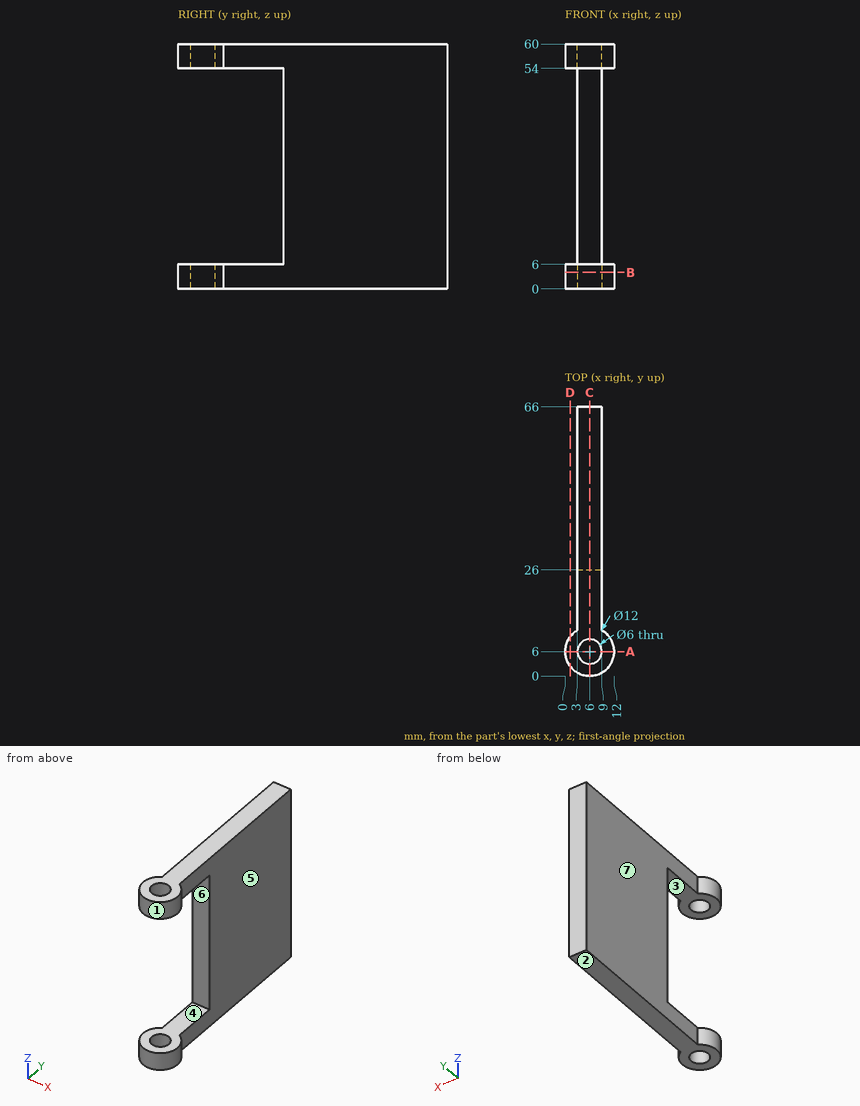
Geometry check sheet. Reference: drawing and pictorial views, mm from the part's lowest x, y, z. A direction names the side the tool comes from. Round coordinates to 2 decimals unless told otherwise and drop trailing zeros. Loops run counter-clockwise (first coordinate to the right, second up) from the corner with the lowest first, then second, coordinate; pieces in that order, holes last.
1. Sectioned sample at C-C on x = 6. Record the boundary of the cut face in (y, z), and give its area (3 significant figures).
2. Sectioned sample at B-B on z = 4. Record the boundary of the cut face in (x, y), and give its area (3 significant figures).
3. Set-up check for the marked faces 5, 6 and 7: record each of +Z, -Z, +X, -X, +Y, -Y from which the full face is reachable in a straight line by a thin tool's end or side.
4. Sectioned sample at A-A on y = 6. Record the boundary of the cut face in (x, z), and give its area (3 significant figures).
5. Sectioned sample at D-D on x = 1.25. Record the boundary of the cut face in (y, z).
6. Gauge pin test, flat ends, axial feed: pin 1 Ø5 at (x, y) = (6, 6) entering from +Z; pin 2 Ø10 at (y, z) = (35.5, 41.5) entering from +X; pin 3 Ø3 at (x, z) = (6, 20) entering from -Y. Record the tip position at first contact, or that the pin passes through.
7. Mould release check, pull along Z, two halves, no side actions. Record for the marked faces 1, 2, 3 and 4: released by +Z, released by -Z, zero draft, split by the parting line, or undercut.
8. Scan lines: probe 1 along Z at (x, y) = (3, 5); probe 2 along Y at (x, z) = (6, 57); probe 3 along X at (y, z) = (41, 37). Record each from-to range of solid material in increasing order.
Recorded:
1. outline: (0, 0) - (3, 0) - (3, 6) - (0, 6) - close; (0, 54) - (3, 54) - (3, 60) - (0, 60) - close; (9, 0) - (66, 0) - (66, 60) - (9, 60) - (9, 54) - (26, 54) - (26, 6) - (9, 6) - close
1. area: 2,640 mm2
2. outline: (3, 11.2) arc R6 ccw (long way) to (9, 11.2) - (9, 66) - (3, 66) - close; hole circle Ø6 at (6, 6)
2. area: 410 mm2
3. face 5: +Z, -Z, +X, +Y
3. face 6: +X, -X, -Y
3. face 7: +Z, -Z, -X, +Y
4. outline: (0, 0) - (3, 0) - (3, 6) - (0, 6) - close; (0, 54) - (3, 54) - (3, 60) - (0, 60) - close; (9, 0) - (12, 0) - (12, 6) - (9, 6) - close; (9, 54) - (12, 54) - (12, 60) - (9, 60) - close
4. area: 72.0 mm2
5. outline: (2.33, 0) - (9.67, 0) - (9.67, 6) - (2.33, 6) - close; (2.33, 54) - (9.67, 54) - (9.67, 60) - (2.33, 60) - close
6. pin 1: passes through
6. pin 2: stops at x = 9
6. pin 3: stops at y = 26
7. face 1: zero draft
7. face 2: released by -Z
7. face 3: undercut
7. face 4: undercut
8. probe 1: z = 0 to 6, 54 to 60
8. probe 2: y = 0 to 3, 9 to 66
8. probe 3: x = 3 to 9
